Can you work these out from the model? Positions are in its coordinate system, mm. Face numbers are marked on the shaded views. Coordinates: 2 decimals unless noted, no trailing zeros. Order: outer loops, then holes, each group sorted by start corner. A loop starts at its lowest first (then second) coordinate and runs counter-clockwise, first axis right, second up. Notation, with made-up numbers: (80, 64.25) -> (122, 64.25) arc R19 cw to (122, 87.25) -> close; hole circle Ø8 at (85, 84). An arc over 180 degrees is marked (long way). Return JSON: item names as keys, results as strings. Group by question number.
1) If we section it at D-D, the plane x = 2.5: Please give me the cut outline in (y, z).
2) For pin 1 (1.5 mm diameter, centred on x = -3, y = 4.5, fed in from +Z); pin 2 (2 mm diameter, centred on x = -3, z = 0, fed in from -Y); pin 3 (1 mm diameter, centred on x = 1.5, z = -3, fed in from +Y), each with a flat end and sliding along its axis, tell me the tip position at first contact or that it passes through.
3) If I drill on probe 1 along Y at (x, z) = (0, 0); probe 2 along Z at (x, y) = (0.25, 0.5); probe 3 along Y at (x, z) = (3.75, 1), over which ranges is the centre line in solid material (lowest first)? Write a range as from..to.
4) If we section it at A-A, the plane y = 0: Please give me the cut outline in (x, z).
5) If we section it at C-C, the plane x = 0.25: Please give me the cut outline in (y, z), then the cut area to 3 significant figures.
6) Thinking about a two-plate mould opening in Y: for the marked faces 1 and 2, which applies, +Y half, -Y half, draft (parallel to the pull), parting line (faces both ways), or undercut?
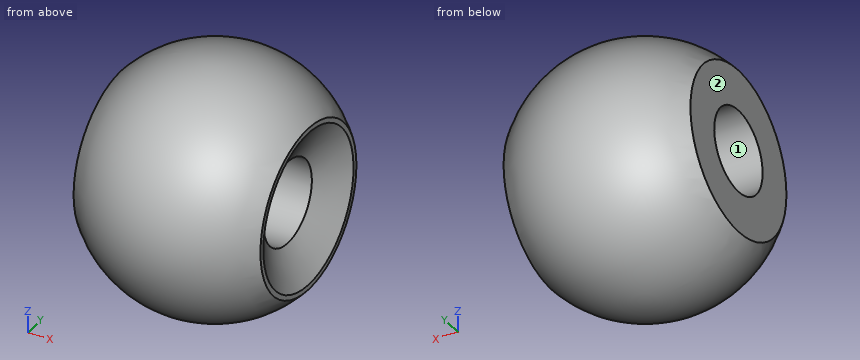
from build123d import *

# Parameters (mm, degrees)
CUT_EXTRUDE1_DEPTH = 10
CUT_EXTRUDE2_REACH = 11
SKETCH4_R          = 2
CHAMFER1_SIZE      = 1
CHAMFER1_SIZE2     = 1.732050808


with BuildPart() as part:
    # Sketch2 → Revolve10 (revolve)
    with BuildSketch(Plane(origin=(0, 0, 0), x_dir=(1, 0, 0), z_dir=(0, 1, 0))):
        with BuildLine():
            Line((0, 6), (0, -6))
            ThreePointArc((0, -6), (-6, 0), (0, 6))
        make_face()
    revolve(axis=Axis((0, 0, -6), (0, 0, 1)))

    # Sketch3 → Cut-Extrude1 (cut, symmetric)
    with BuildSketch(Plane(origin=(0, 0, 0), x_dir=(1, 0, 0), z_dir=(0, 1, 0))):
        Polygon((-4.5, 6.116617365), (-8.039926199, -0.619090826), (-4.5, -6.116617365), align=None)
        Polygon((4.5, -6.116617365), (4.5, 6.116617365), (7.115417232, -1.229927109), align=None)
    extrude(amount=CUT_EXTRUDE1_DEPTH, both=True, mode=Mode.SUBTRACT)

    # Sketch4 → Cut-Extrude2 (cut, up to next)
    with BuildSketch(Plane(origin=(4.5, 0, 0), x_dir=(0, 0, -1), z_dir=(1, 0, 0)), mode=Mode.PRIVATE) as cut_extrude2_sk1:
        Circle(SKETCH4_R)
    cut_extrude2_tool1 = extrude(cut_extrude2_sk1.sketch, amount=-CUT_EXTRUDE2_REACH, mode=Mode.PRIVATE) & part.part
    add(cut_extrude2_tool1.solids().sort_by_distance((4.5, 0, 0))[0], mode=Mode.SUBTRACT)

    # Chamfer1
    chamfer1_edges = [part.edges().sort_by_distance(p)[0] for p in [
        (4.5, 0, 2),
    ]]
    chamfer1_side = [part.faces().sort_by_distance(p)[0] for p in [
        (0, 0, 2),
    ]]
    chamfer(chamfer1_edges, length=CHAMFER1_SIZE, length2=CHAMFER1_SIZE2, reference=chamfer1_side[0])


solid = part.part
Result sheet:
{
 "1": {"outline": "circle Ø10.91 at (0, 0); hole circle Ø4 at (0, 0)"},
 "2": {"pin 1": "stops at z = 3.78", "pin 2": "stops at y = -5.66", "pin 3": "stops at y = 5.28"},
 "3": {"probe 1": "y = -6..-2, 2..6", "probe 2": "z = -5.97..-1.94, 1.94..5.97", "probe 3": "y = -4.58..-2.22, 2.22..4.58"},
 "4": {"outline": "(-4.5, -3.97) arc R6 ccw to (4.5, -3.97) -> (4.5, -3.73) -> (3.5, -2) -> (-4.5, -2) -> close; (-4.5, 2) -> (3.5, 2) -> (4.5, 3.73) -> (4.5, 3.97) arc R6 ccw to (-4.5, 3.97) -> close"},
 "5": {"outline": "circle Ø11.99 at (0, 0); hole circle Ø4 at (0, 0)", "area": "100 mm2"},
 "6": {"face 1": "undercut", "face 2": "draft"}
}
